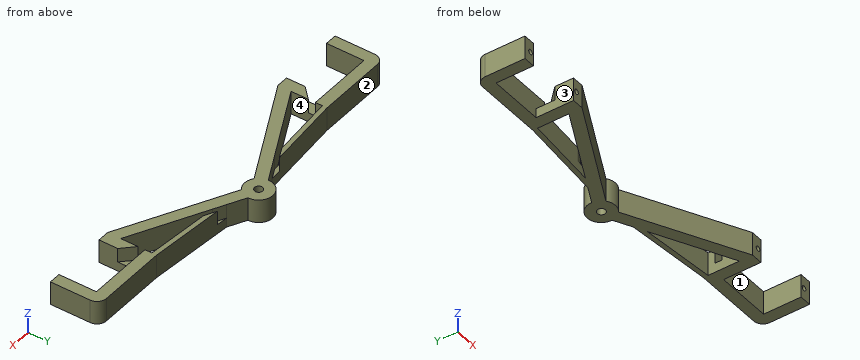
```python
from build123d import *

# Parameters (mm, degrees)
SKICA1_R                 = 1.75
P_IDAT_VYSUNUT_M1_DEPTH  = 5
ZAOBLIT1_R               = 4
P_IDAT_VYSUNUT_M2_DEPTH  = 5
SKICA3_R                 = 1.05
ODEBRAT_VYSUNUT_M1_DEPTH = 6
ODEBRAT_VYSUNUT_M2_DEPTH = 6
ODEBRAT_VYSUNUT_M3_DEPTH = 6


with BuildPart() as part:
    # Skica1 → Přidat vysunutím1 (new body, symmetric)
    with BuildSketch(Plane.XY):
        with BuildLine():
            Line((0, 0), (0, 16))
            Line((0, 16), (23.5, 16))
            Line((23.5, 16), (23.5, 0))
            Line((23.5, 0), (28.5, 0))
            Line((28.5, 0), (74.768828107, 23.497329584))
            ThreePointArc((74.768828107, 23.497329584), (78.5, 22.196090729), (82.231171893, 23.497329584))
            Line((82.231171893, 23.497329584), (128.5, 0))
            Line((128.5, 0), (133.5, 0))
            Line((133.5, 0), (133.5, 16))
            Line((133.5, 16), (157, 16))
            Line((157, 16), (157, 0))
            Line((157, 0), (162, 0))
            Line((162, 0), (162, 21))
            Line((162, 21), (128.5, 21))
            Line((128.5, 21), (128.5, 5.607818541))
            Line((128.5, 5.607818541), (84.49517003, 27.955391095))
            ThreePointArc((84.49517003, 27.955391095), (78.5, 34.196090729), (72.50482997, 27.955391095))
            Line((72.50482997, 27.955391095), (28.5, 5.607818541))
            Line((28.5, 5.607818541), (28.5, 21))
            Line((28.5, 21), (-5, 21))
            Line((-5, 21), (-5, 0))
            Line((-5, 0), (0, 0))
        make_face()
        with Locations((78.5, 28.196090729)):
            Circle(SKICA1_R, mode=Mode.SUBTRACT)
    extrude(amount=P_IDAT_VYSUNUT_M1_DEPTH, both=True)

    # Zaoblit1
    zaoblit1_edges = [part.edges().sort_by_distance(p)[0] for p in [
        (-5, 21, 0),
        (162, 21, 0),
    ]]
    fillet(zaoblit1_edges, radius=ZAOBLIT1_R)

    # Skica2 → Přidat vysunutím2 (add, symmetric)
    with BuildSketch(Plane.XY):
        Polygon((28.5, 21), (65.117103916, 24.203581484), (60.341045967, 21.778090882), (28.5, 18.992360325), align=None)
    p_idat_vysunut_m2 = extrude(amount=P_IDAT_VYSUNUT_M2_DEPTH, both=True)

    # Zrcadlit1: Přidat vysunutím2 across plane
    add(p_idat_vysunut_m2.mirror(Plane.ZY.offset(-78.5)))

    # Skica3 → Odebrat vysunutím1 (cut)
    with BuildSketch(Plane.XZ):
        with Locations((-1.75, 0)):
            Circle(SKICA3_R)
        with Locations((25.25, 0)):
            Circle(SKICA3_R)
    odebrat_vysunut_m1 = extrude(amount=-ODEBRAT_VYSUNUT_M1_DEPTH, mode=Mode.SUBTRACT)

    # Zrcadlit2: Odebrat vysunutím1 across plane
    add(odebrat_vysunut_m1.mirror(Plane.ZY.offset(-78.5)), mode=Mode.SUBTRACT)

    # Skica4 → Odebrat vysunutím2 (cut)
    with BuildSketch(Plane.XY.offset(5)):
        Polygon((23.5, 16), (28.5, 16), (28.5, 13), (23.5, 8), align=None)
    odebrat_vysunut_m2 = extrude(amount=-ODEBRAT_VYSUNUT_M2_DEPTH, mode=Mode.SUBTRACT)

    # Zrcadlit3: Odebrat vysunutím2 across plane
    add(odebrat_vysunut_m2.mirror(Plane.ZY.offset(-78.5)), mode=Mode.SUBTRACT)

    # Skica5 → Odebrat vysunutím3 (cut)
    with BuildSketch(Plane.XY.offset(5)):
        Polygon((60.341045967, 21.778090882), (65.117103916, 24.203581484), (60.314461293, 23.783404699), (55.538403344, 21.357914097), align=None)
        Polygon((91.882896084, 24.203581484), (96.685538707, 23.783404699), (101.461596656, 21.357914097), (96.658954033, 21.778090882), align=None)
    extrude(amount=-ODEBRAT_VYSUNUT_M3_DEPTH, mode=Mode.SUBTRACT)


solid = part.part
```
Geometry check sheet. Reference: the model listing, model coordinates, mm. Face numbers are marked on the shaded views. A direction names the side the tool comes from. Coordinates: 2 decimals unless noted, no trailing zeros. Order: outer loops, then holes, each group sorted by start corner. A loop starts at its lowest first (then second) coordinate and runs counter-clockwise, first axis right, second up. Notation, with made-up numbers: (-32.5, -24) - (-2.5, -24) arc R11 ccw to (-2.5, -19) - close; hole circle Ø1 at (1.25, 78.25). An arc over 180 degrees is marked (long way). Answer as a JSON object with one key per item and string values. Group by question number.
Item 1: Sectioned sample at D-D, the plane x = 143. Record the cut outline in (y, z), and give its area (3 significant figures).
Item 2: Depth check by flat-ended pin: pin 1 Ø3.5 at (x, z) = (158.75, 0) entering from -Y; pin 2 Ø2.5 at (x, z) = (-1.75, 0) entering from +Y; pin 3 Ø5 at (x, z) = (139.5, 1.5) entering from -Y. Enter the tip coordinate at first touch or a pass-through.
Item 3: Scan lines: probe 1 along Z at (x, y) = (25.25, 1.6); probe 2 along X at (y, z) = (17, 0.5); probe 3 along X at (y, z) = (13.5, -0.25). Record each from-to range of solid material in increasing order.
Item 4: Sectioned sample at A-A, the plane x = 78.5. Record the cut outline in (y, z).
Item 5: Tool access check on the marked faces 1, 2, 3 and 4. Record the directions out of +Z, -Z, +X, -X, +Y, -Y that give a thin tool (end or side, any length) a straight path to the whole face; none if there is none.
Item 6: Sectioned sample at C-C, the plane z = -2.5. Give the number of separate pieces and of enclosed holes in the cut face, and give its area (3 significant figures).
Item 7: Sectioned sample at B-B, the plane y = 4. Record the cut outline in (x, z), and give its area (3 significant figures).
Resolved:
{
 "1": {"outline": "(16, -5) - (21, -5) - (21, 5) - (16, 5) - close", "area": "50.0 mm^2"},
 "2": {"pin 1": "y = 0", "pin 2": "y = 21", "pin 3": "y = 16"},
 "3": {"probe 1": "-5 to -1.05, 1.05 to 5", "probe 2": "-5 to 28.5, 50.93 to 61.97, 95.03 to 106.07, 128.5 to 162", "probe 3": "-5 to 0, 44.04 to 55.08, 101.92 to 112.96, 157 to 162"},
 "4": {"outline": "(22.2, -5) - (26.45, -5) - (26.45, 5) - (22.2, 5) - close; (29.95, -5) - (34.2, -5) - (34.2, 5) - (29.95, 5) - close"},
 "5": {"face 1": "+Z", "face 2": "+Z, -Z, -X, +Y", "face 3": "+Z, -Z, -Y", "face 4": "+Z, -Z"},
 "6": {"separate pieces": "1", "enclosed holes": "3", "area": "1,390 mm^2"},
 "7": {"outline": "(-5, -5) - (0, -5) - (0, 5) - (-5, 5) - close; (23.5, -5) - (36.38, -5) - (36.38, 5) - (23.5, 5) - close; (120.62, -5) - (133.5, -5) - (133.5, 5) - (120.62, 5) - close; (157, -5) - (162, -5) - (162, 5) - (157, 5) - close; hole circle Ø2.1 at (-1.75, 0); hole circle Ø2.1 at (25.25, 0); hole circle Ø2.1 at (131.75, 0); hole circle Ø2.1 at (158.75, 0)", "area": "344 mm^2"}
}
